from build123d import *

# Parameters (mm, degrees)
F1_DEPTH  = 1000
F3_DEPTH  = 550
F2_W      = 75
F2_H      = 75
F5_DEPTH  = 315
F6_W      = 550
F6_H      = 300
F6_R      = 6
F7_DEPTH  = 16
F9_W      = 190
F9_H      = 75
F9_R      = 5
F10_DEPTH = 12
F12_W     = 100
F12_H     = 75
F14_DEPTH = 6
F16_R     = 3
F17_DEPTH = 12
F18_W     = 65
F18_H     = 65
F19_DEPTH = 9
F21_W     = 65
F21_H     = 65
F22_DEPTH = 9
F23_R     = 5
F23_R_2   = 15
F24_DEPTH = 25
F25_R     = 5
F25_R_2   = 15
F26_DEPTH = 25


with BuildPart() as f1:
    # F0 (on Front) → F1 (new body)
    with BuildSketch(Plane.XZ):
        Polygon((40, 0), (0, 0), (0, -75), (40, -75), (40, -70), (5, -70), (5, -5), (40, -5), align=None)
    extrude(amount=F1_DEPTH)


with BuildPart() as f1b:
    # F0 (on Front) → F1, piece 2 (new body)
    with BuildSketch(Plane.XZ):
        Polygon((545, -70), (510, -70), (510, -75), (550, -75), (550, 0), (510, 0), (510, -5), (545, -5), align=None)
    extrude(amount=F1_DEPTH)


with BuildPart() as f1c:
    # F0 (on Front) → F1, piece 3 (new body)
    with BuildSketch(Plane.XZ):
        Polygon((40, -390), (0, -390), (0, -465), (40, -465), (40, -460), (5, -460), (5, -395), (40, -395), align=None)
    extrude(amount=F1_DEPTH)


with BuildPart() as f1d:
    # F0 (on Front) → F1, piece 4 (new body)
    with BuildSketch(Plane.XZ):
        Polygon((545, -460), (510, -460), (510, -465), (550, -465), (550, -390), (510, -390), (510, -395), (545, -395), align=None)
    extrude(amount=F1_DEPTH)


with BuildPart() as f3:
    # F2 (on Right) → F3 (new body)
    with BuildSketch(Plane.YZ):
        Polygon((-40, -75), (0, -75), (0, 0), (-40, 0), (-40, -5), (-5, -5), (-5, -70), (-40, -70), align=None)
    extrude(amount=F3_DEPTH)


with BuildPart() as f3b:
    # F2 (on Right) → F3, piece 2 (new body)
    with BuildSketch(Plane.YZ):
        Polygon((-960, -5), (-960, 0), (-1000, 0), (-1000, -75), (-960, -75), (-960, -70), (-995, -70), (-995, -5), align=None)
    extrude(amount=F3_DEPTH)

    # F9 (on offset) → F10 (join)
    with BuildSketch(Plane.XZ.offset(1000)):
        with Locations((275, -37.5)):
            Rectangle(F9_W, F9_H)
        with Locations((225, -55)):
            Circle(F9_R, mode=Mode.SUBTRACT)
        with Locations((325, -55)):
            Circle(F9_R, mode=Mode.SUBTRACT)
        with Locations((225, -20)):
            Circle(F9_R, mode=Mode.SUBTRACT)
        with Locations((325, -20)):
            Circle(F9_R, mode=Mode.SUBTRACT)
    extrude(amount=F10_DEPTH)


with BuildPart() as f3c:
    # F2 (on Right) → F3, piece 3 (new body)
    with BuildSketch(Plane.YZ):
        Polygon((-240, -40), (-235, -40), (-235, 0), (-310, 0), (-310, -40), (-305, -40), (-305, -5), (-240, -5), align=None)
    extrude(amount=F3_DEPTH)


with BuildPart() as f3d:
    # F2 (on Right) → F3, piece 4 (new body)
    with BuildSketch(Plane.YZ):
        Polygon((-960, -395), (-960, -390), (-1000, -390), (-1000, -465), (-960, -465), (-960, -460), (-995, -460), (-995, -395), align=None)
    extrude(amount=F3_DEPTH)


with BuildPart() as f3e:
    # F2 (on Right) → F3, piece 5 (new body)
    with BuildSketch(Plane.YZ):
        with Locations((-37.5, -427.5)):
            Rectangle(F2_W, F2_H)
    extrude(amount=F3_DEPTH)


with BuildPart() as f5:
    # F4 (on face) → F5 (new body)
    with BuildSketch(Plane.XY.offset(-390)):
        Polygon((0, -925), (0, -1000), (40, -1000), (40, -995), (5, -995), (5, -930), (40, -930), (40, -925), align=None)
    extrude(amount=F5_DEPTH)


with BuildPart() as f5b:
    # F4 (on face) → F5, piece 2 (new body)
    with BuildSketch(Plane.XY.offset(-390)):
        Polygon((545, -995), (510, -995), (510, -1000), (550, -1000), (550, -925), (510, -925), (510, -930), (545, -930), align=None)
    extrude(amount=F5_DEPTH)


with BuildPart() as f5c:
    # F4 (on face) → F5, piece 3 (new body)
    with BuildSketch(Plane.XY.offset(-390)):
        Polygon((0, 0), (0, -75), (40, -75), (40, -70), (5, -70), (5, -5), (40, -5), (40, 0), align=None)
    extrude(amount=F5_DEPTH)


with BuildPart() as f5d:
    # F4 (on face) → F5, piece 4 (new body)
    with BuildSketch(Plane.XY.offset(-390)):
        Polygon((545, -70), (510, -70), (510, -75), (550, -75), (550, 0), (510, 0), (510, -5), (545, -5), align=None)
    extrude(amount=F5_DEPTH)


with BuildPart() as f7:
    # F6 (on Top) → F7 (new body)
    with BuildSketch(Plane.XY):
        with Locations((275, -150)):
            Rectangle(F6_W, F6_H)
        with Locations((150, -270.8259150982)):
            Circle(F6_R, mode=Mode.SUBTRACT)
        with Locations((400, -270.8259150982)):
            Circle(F6_R, mode=Mode.SUBTRACT)
        with Locations((150, -134.8259150982)):
            Circle(F6_R, mode=Mode.SUBTRACT)
        with Locations((400, -134.8259150982)):
            Circle(F6_R, mode=Mode.SUBTRACT)
    extrude(amount=F7_DEPTH)


with BuildPart() as f1_1:
    add(f1.part)

    # F13: union F1b, F1c, F1d, F3, F3d, F5b, F7, F3b, F3c, F3e, F5, F5c, F5d
    add(f1b.part)
    add(f1c.part)
    add(f1d.part)
    add(f3.part)
    add(f3d.part)
    add(f5b.part)
    add(f7.part)
    add(f3b.part)
    add(f3c.part)
    add(f3e.part)
    add(f5.part)
    add(f5c.part)
    add(f5d.part)

    # F12 (on offset) → F14 (join)
    with BuildSketch(Plane(origin=(0, 0, -465), x_dir=(1, 0, 0), z_dir=(0, 0, -1))):
        with Locations((165, 37.5)):
            Rectangle(F12_W, F12_H)
        with Locations((385, 37.5)):
            Rectangle(F12_W, F12_H)
        with Locations((165, 962.5)):
            Rectangle(F12_W, F12_H)
        with Locations((385, 962.5)):
            Rectangle(F12_W, F12_H)
    extrude(amount=F14_DEPTH)

    # F16 (on offset) → F17 (cut)
    with BuildSketch(Plane(origin=(0, 0, -471), x_dir=(1, 0, 0), z_dir=(0, 0, -1))):
        with Locations((407.5, 934)):
            Circle(F16_R)
        with Locations((407.5, 991)):
            Circle(F16_R)
        with Locations((362.5, 991)):
            Circle(F16_R)
        with Locations((362.5, 934)):
            Circle(F16_R)
        with Locations((407.5, 9)):
            Circle(F16_R)
        with Locations((407.5, 66)):
            Circle(F16_R)
        with Locations((362.5, 66)):
            Circle(F16_R)
        with Locations((362.5, 9)):
            Circle(F16_R)
        with Locations((174.8421853781, 934)):
            Circle(F16_R)
        with Locations((174.8421853781, 991)):
            Circle(F16_R)
        with Locations((129.8421853781, 991)):
            Circle(F16_R)
        with Locations((129.8421853781, 934)):
            Circle(F16_R)
        with Locations((174.8421853781, 9)):
            Circle(F16_R)
        with Locations((174.8421853781, 66)):
            Circle(F16_R)
        with Locations((129.8421853781, 66)):
            Circle(F16_R)
        with Locations((129.8421853781, 9)):
            Circle(F16_R)
    extrude(amount=-F17_DEPTH, mode=Mode.SUBTRACT)

    # F18 (on Right) → F19 (join)
    with BuildSketch(Plane.YZ):
        with Locations((-745, -423.5)):
            Rectangle(F18_W, F18_H)
    extrude(amount=-F19_DEPTH)

    # F21 (on offset) → F22 (join)
    with BuildSketch(Plane.YZ.offset(550)):
        with Locations((-745, -423.5)):
            Rectangle(F21_W, F21_H)
    extrude(amount=F22_DEPTH)

    # F23 (on face) → F24 (cut)
    with BuildSketch(Plane.YZ.offset(559)):
        with Locations((-764.5, -406)):
            Circle(F23_R)
        with Locations((-724.5, -406)):
            Circle(F23_R)
        with Locations((-744.5, -436)):
            Circle(F23_R_2)
    extrude(amount=-F24_DEPTH, mode=Mode.SUBTRACT)

    # F25 (on face) → F26 (cut)
    with BuildSketch(Plane(origin=(-9, 0, 0), x_dir=(0, -1, 0), z_dir=(-1, 0, 0))):
        with Locations((725.5, -407)):
            Circle(F25_R)
        with Locations((765.5, -407)):
            Circle(F25_R)
        with Locations((745.5, -437)):
            Circle(F25_R_2)
    extrude(amount=-F26_DEPTH, mode=Mode.SUBTRACT)


solid = f1_1.part
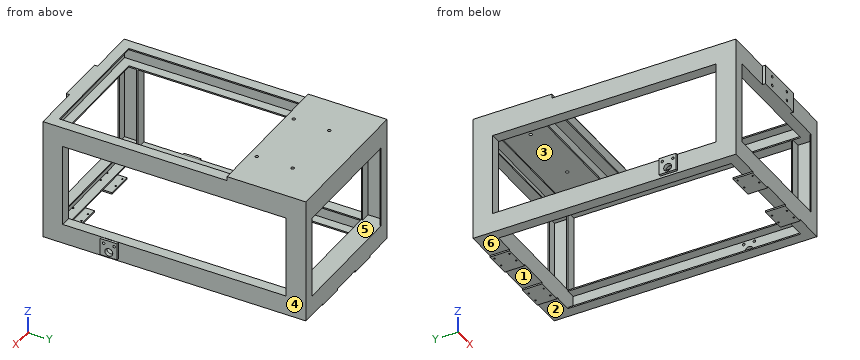
Input: part model. Units: mm. Frame: model coordinates. Face numbers are marked on the shaded views. A direction names the side the tool comes from. Coordinates: 2 decimals unless noted, no trailing zeros. Write item = value, one per line. Start each with the question number.
Item 1: Mould query, pull axis Z, two halves, no side actions, for the marked faces 4, 5 and 6. Classes: pulls with the +Z half, pulls with the -Z half, needs draft (parallel to the pull), parting line crosses it, or undercut.
Item 2: Material intervals for line 1 (Y direction, x = 511, z = -205); line 2 (X direction, y = -991, z = -463); line 3 (Y direction, x = 407.5, z = -463), sorted ascending.
Item 3: Reachability of the marked faces 1, 2 and 3 from +Z, -Z, +X, -X, +Y, -Y: full face, straight path, thin tool, end or side. Return the list, or none.
Item 4: First-contact query: P1, Ø5, axis at x = 130, y = -66, coming from the -Z side; P2, Ø2.5, axis at x = -4.5, z = -439.5, coming from the -Y side; P3, Ø5.5, axis at x = 129.84, y = -991, coming from the +Z side. Flat tips, straight axial feed; report the tip coordinate or a pass-through.
Item 5: Cut plane A-A, the plane y = -908.5. Count the separate pieces of the cut face and the enclosed holes in it, plus the area to 3 significant figures.
Ans:
q1.face_4 = needs draft
q1.face_5 = undercut
q1.face_6 = pulls with the -Z half
q2.line_1 = -1000 to -995, -930 to -925, -75 to -70, -5 to 0
q2.line_2 = 0 to 126.84, 132.84 to 171.84, 177.84 to 359.5, 365.5 to 404.5, 410.5 to 550
q2.line_3 = -1000 to -994, -988 to -960, -75 to -69, -63 to -12, -6 to 0
q3.face_1 = -Z, +Y, -Y
q3.face_2 = -Z, +X, +Y, -Y
q3.face_3 = none
q4.P1 = -459
q4.P2 = -777.5
q4.P3 = 0
q5.separate_pieces = 4
q5.enclosed_holes = 0
q5.area = 2,900 mm²
